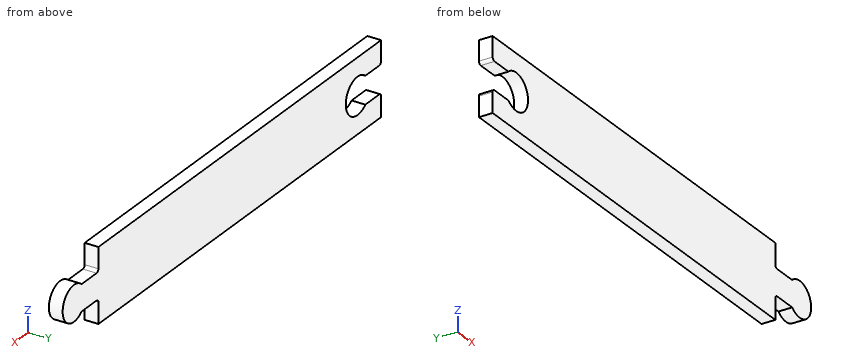
```python
from build123d import *

# Parameters (mm, degrees)
BOSS_EXTRUDE1_DEPTH = 4.7625
FILLET1_R           = 1


with BuildPart() as part:
    # Sketch1 → Boss-Extrude1 (new body)
    with BuildSketch(Plane(origin=(0, 0, 0), x_dir=(1, 0, 0), z_dir=(0, 1, 0))):
        with BuildLine():
            Line((-76.2, -12.7), (76.2, -12.7))
            Line((76.2, -12.7), (76.2, -4.5125))
            Line((76.2, -4.5125), (85.295448411, -4.5125))
            ThreePointArc((85.295448411, -4.5125), (95.5, 0), (85.295448411, 4.5125))
            Line((85.295448411, 4.5125), (76.2, 4.5125))
            Line((76.2, 4.5125), (76.2, 12.7))
            Line((76.2, 12.7), (-76.2, 12.7))
            Line((-76.2, 12.7), (-76.2, 4.7625))
            Line((-76.2, 4.7625), (-67.700130206, 4.7625))
            ThreePointArc((-67.700130206, 4.7625), (-57.15, 0), (-67.700130206, -4.7625))
            Line((-67.700130206, -4.7625), (-76.2, -4.7625))
            Line((-76.2, -4.7625), (-76.2, -12.7))
        make_face()
    extrude(amount=BOSS_EXTRUDE1_DEPTH)

    # Fillet1
    fillet1_edges = [part.edges().sort_by_distance(p)[0] for p in [
        (76.2, 2.38125, -4.5125),
        (76.2, 2.38125, 4.5125),
        (-76.2, 2.38125, 4.7625),
        (-76.2, 2.38125, -4.7625),
    ]]
    fillet(fillet1_edges, radius=FILLET1_R)


solid = part.part
```
Model file for the job. Use its own axes, mm. Coordinates: 2 decimals unless noted, no trailing zeros. Write each loop counter-clockwise with the first axis right and the second up, starting at its lowest first coordinate (ties: lowest second). Pieces come first, ordered by that corner, then holes. Notation, with made-up numbers: (-38.5, 88.25) - (16.5, 88.25) arc R15 cw to (16.5, 93.25) - close; hole circle Ø11 at (83, 49). An arc over 180 degrees is marked (long way). One line per question, with ' | ' between items. Start each with the question number.
Q1. Cut at D-D, the plane x = 79.5. List the corners of the cut face in (y, z).
Q2. Cut at B-B, the plane y = 3.3. List the corners of the cut face in (x, z), then the cut area to 3 significant figures.
Q3. Cut at C-C, the plane z = 0. List the corners of the cut face in (x, y).
Q4. Cut at A-A, the plane x = -63.5. List the corners of the cut face in (y, z).
Q5. Drill centre lines: line 1 (Z direction, x = -63.5, y = 1.05); line 2 (X direction, y = 4.5, z = -7.25); line 3 (X direction, y = 2.7, z = 2.75). Where is each one in solid material? Low to high. Write a range as [from, to].
Q6. Pin check, flat tips, straight feed: pin 1 (1.4 mm diameter, centred on x = 80.5, y = 2.5, fed in from +Z); pin 2 (2.5 mm diameter, centred on x = 79, y = 3.5, fed in from -Z); pin 3 (1.4 mm diameter, centred on y = 1.5, z = 10, fed in from +X). Stop position of each tip, or through.
Answer below:
1) outline: (0, -4.51) - (4.76, -4.51) - (4.76, 4.51) - (0, 4.51) - close
2) outline: (-76.2, -12.7) - (76.2, -12.7) - (76.2, -5.51) arc R1 cw to (77.2, -4.51) - (85.3, -4.51) arc R6.1 ccw (long way) to (85.3, 4.51) - (77.2, 4.51) arc R1 cw to (76.2, 5.51) - (76.2, 12.7) - (-76.2, 12.7) - (-76.2, 5.76) arc R1 ccw to (-75.2, 4.76) - (-67.7, 4.76) arc R6.35 cw (long way) to (-67.7, -4.76) - (-75.2, -4.76) arc R1 ccw to (-76.2, -5.76) - close | area: 3,860 mm^2
3) outline: (-57.15, 0) - (95.5, 0) - (95.5, 4.76) - (-57.15, 4.76) - close
4) outline: (0, -12.7) - (4.76, -12.7) - (4.76, -6.35) - (0, -6.35) - close; (0, 6.35) - (4.76, 6.35) - (4.76, 12.7) - (0, 12.7) - close
5) line 1: [-12.7, -6.35], [6.35, 12.7] | line 2: [-76.2, 76.2] | line 3: [-57.78, 94.84]
6) pin 1: z = 4.51 | pin 2: z = -4.51 | pin 3: x = 76.2
